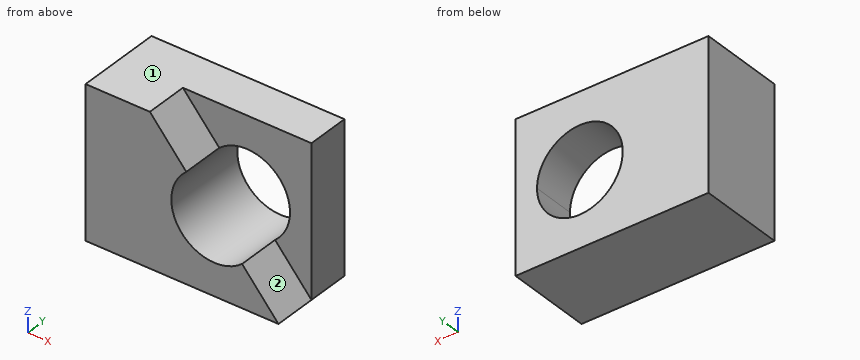
```python
from build123d import *

# Parameters (mm, degrees)
F0_W     = 12.7
F0_H     = 44.45
F1_DEPTH = 57.15
F3_DEPTH = 12.7
F5_DEPTH = 25.4


with BuildPart() as f1:
    # F0 (on Right) → F1 (new body)
    with BuildSketch(Plane.YZ):
        with Locations((6.35, 22.225)):
            Rectangle(F0_W, F0_H)
    extrude(amount=F1_DEPTH)

    # F2 (on face) → F3 (join)
    with BuildSketch(Plane.XZ):
        Polygon((0, 44.45), (0, 0), (57.15, 0), (19.05, 44.45), align=None)
    extrude(amount=F3_DEPTH)

    # F4 (on face) → F5 (cut)
    with BuildSketch(Plane.XZ.offset(12.7)):
        with BuildLine():
            Line((46.36505, 12.582441), (29.83495, 31.867559))
            ThreePointArc((29.83495, 31.867559), (28.457441, 13.95995), (46.36505, 12.582441))
        make_face()
        with BuildLine():
            ThreePointArc((46.36505, 12.582441), (49.638114, 16.918219), (50.8, 22.225))
            ThreePointArc((50.8, 22.225), (43.406781, 33.763114), (29.83495, 31.867559))
            Line((29.83495, 31.867559), (46.36505, 12.582441))
        make_face()
    extrude(amount=-F5_DEPTH, mode=Mode.SUBTRACT)


solid = f1.part
```
CAD build for the part. Positions are in the model's coordinates, mm. Face numbers are marked on the shaded views. A direction names the side the tool comes from. Round coordinates to 2 decimals unless told otherwise and drop trailing zeros. Order: outer loops, then holes, each group sorted by start corner. A loop starts at its lowest first (then second) coordinate and runs counter-clockwise, first axis right, second up. Notation, with made-up numbers: (60.5, 23.25) - (102.5, 23.25) arc R31 ccw to (102.5, 50.25) - close; hole circle Ø9 at (61.5, 55.5). An arc over 180 degrees is marked (long way). Answer as CSV lines item,"result". Start each with the question number.
1. Saw through at D-D, the plane y = -2.5. Write the cut outline in (x, z) (3 decimals).
2. Tool access for the marked faces 1 and 2: list every direction of +Z, -Z, +X, -X, +Y, -Y with a clear straight run to the whole face (end or side of a thin tool).
3. Saw through at C-C, the plane z = 30.5. Write the cut outline in (x, y).
4. Saw through at A-A, the plane y = 5.75. Write the cut outline in (x, z) (3 decimals).
5. Drill centre lines: L1, parallel to Y at x = 27, z = 41.5; L2, parallel to Z at x = 44.5, y = 9.5; L3, parallel to Z at x = 48, y = 7. Where is each one in solid material? Low to high. Write a range as [from, to].
6. Saw through at B-B, the plane x = 38.1. Write the cut outline in (y, z) (3 decimals).
Model answer:
1,outline,"(0, 0) - (57.15, 0) - (46.365, 12.582) arc R12.7 cw to (29.835, 31.868) - (19.05, 44.45) - (0, 44.45) - close"
2,face 1,"+Z, +X, -X, +Y, -Y"
2,face 2,"+Z, +X, -Y"
3,outline,"(0, -12.7) - (28.47, -12.7) - (28.47, 12.7) - (0, 12.7) - close; (47.73, 0) - (57.15, 0) - (57.15, 12.7) - (47.73, 12.7) - close"
4,outline,"(0, 0) - (57.15, 0) - (57.15, 44.45) - (0, 44.45) - close; hole circle Ø25.4 at (38.1, 22.225)"
5,L1,"y = [0, 12.7]"
5,L2,"z = [0, 11.26], [33.19, 44.45]"
5,L3,"z = [0, 14.27], [30.18, 44.45]"
6,outline,"(-12.7, 0) - (12.7, 0) - (12.7, 9.525) - (-12.7, 9.525) - close; (0, 34.925) - (12.7, 34.925) - (12.7, 44.45) - (0, 44.45) - close"
